For this review, take the finished solid that the model builds, in its own axes (mm). Coordinates: 2 decimals unless noted, no trailing zeros. Loops run counter-clockwise (first coordinate to the right, second up) from the corner with the lowest first, then second, coordinate; pieces in that order, holes last. Notation, with made-up numbers: (20, 64) -> (69, 64) arc R19 cw to (69, 95) -> close; hole circle Ø2 at (55.25, 64). An arc over 180 degrees is marked (long way). One line per item, written item: value.
from build123d import *

# Parameters (mm, degrees)
CROQUIS1_W              = 111
CROQUIS1_H              = 86.5
CROQUIS1_W_2            = 7.783251258
CROQUIS1_H_2            = 10.118226634
SALIENTE_EXTRUIR1_DEPTH = 5
CROQUIS3_W              = 111
CROQUIS3_H              = 5
SALIENTE_EXTRUIR2_DEPTH = 6


with BuildPart() as part:
    # Croquis1 → Saliente-Extruir1 (new body)
    with BuildSketch(Plane.XY):
        with Locations((50.205582562, 38.585714286)):
            Rectangle(CROQUIS1_W, CROQUIS1_H)
        Polygon((-1.339906851, 59.600947476), (4.653483533, 65.703308594), (73.52298758, 65.703308594), (73.52298758, 59.600947476), (6.614956749, 59.600947476), (6.614956749, 17.756185524), (81.586821915, 17.756185524), (81.586821915, 11), (6.614956749, 11), (-1.339906851, 11), align=None, mode=Mode.SUBTRACT)
        Polygon((29.151946634, 43.268500853), (37.324360454, 43.268500853), (37.324360454, 51.311193819), (61.582160207, 51.311193819), (61.582160207, 25.756185524), (37.324360454, 25.756185524), (37.324360454, 30.945019695), (29.151946634, 30.945019695), align=None, mode=Mode.SUBTRACT)
        with Locations((73.516478802, 50.815298841)):
            Rectangle(CROQUIS1_W_2, CROQUIS1_H_2, mode=Mode.SUBTRACT)
    extrude(amount=SALIENTE_EXTRUIR1_DEPTH)

    # Croquis3 → Saliente-Extruir2 (add)
    with BuildSketch(Plane(origin=(0, 81.835714286, 0), x_dir=(1, 0, 0), z_dir=(0, 1, 0))):
        with Locations((50.205582562, -2.5)):
            Rectangle(CROQUIS3_W, CROQUIS3_H)
    extrude(amount=SALIENTE_EXTRUIR2_DEPTH)


solid = part.part
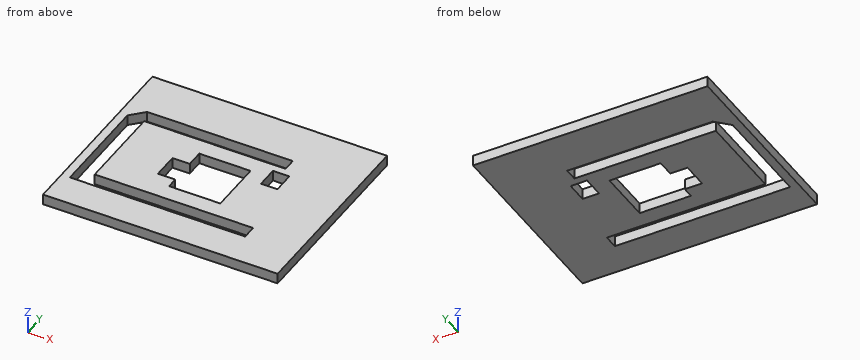
1. Take a section at D-D, the plane y = 23. Give the boundary of the cut face in (x, z).
Return value:
outline: (-5.29, 0) -> (-1.34, 0) -> (-1.34, 5) -> (-5.29, 5) -> close; (6.61, 0) -> (105.71, 0) -> (105.71, 5) -> (6.61, 5) -> close
2. Take a section at B-B, the plane x = 43.5. Give the boundary of the cut face in (y, z).
Return value:
outline: (-4.66, 0) -> (11, 0) -> (11, 5) -> (-4.66, 5) -> close; (17.76, 0) -> (25.76, 0) -> (25.76, 5) -> (17.76, 5) -> close; (51.31, 0) -> (59.6, 0) -> (59.6, 5) -> (51.31, 5) -> close; (65.7, 0) -> (87.84, 0) -> (87.84, 5) -> (65.7, 5) -> close
3. To check wall thickness, follow probe 1 along Y at (x, z) = (65.5, 0.3); probe 2 along Y at (x, z) = (41.5, 3.65); probe 3 along Y at (x, z) = (72, 1.5). State the ranges of each line that lie inside material, in increasing order. Write a range as from..to.
Return value:
probe 1: y = -4.66..11, 17.76..59.6, 65.7..87.84
probe 2: y = -4.66..11, 17.76..25.76, 51.31..59.6, 65.7..87.84
probe 3: y = -4.66..11, 17.76..45.76, 55.87..59.6, 65.7..87.84
4. Take a section at C-C, the plane z = 2.4. Give the boundary of the cut face in (x, y), and give its area (3 significant figures).
Return value:
outline: (-5.29, -4.66) -> (105.71, -4.66) -> (105.71, 87.84) -> (-5.29, 87.84) -> close; hole (-1.34, 11) -> (81.59, 11) -> (81.59, 17.76) -> (6.61, 17.76) -> (6.61, 59.6) -> (73.52, 59.6) -> (73.52, 65.7) -> (4.65, 65.7) -> (-1.34, 59.6) -> close; hole (29.15, 30.95) -> (37.32, 30.95) -> (37.32, 25.76) -> (61.58, 25.76) -> (61.58, 51.31) -> (37.32, 51.31) -> (37.32, 43.27) -> (29.15, 43.27) -> close; hole (69.62, 45.76) -> (77.41, 45.76) -> (77.41, 55.87) -> (69.62, 55.87) -> close
area: 8,140 mm2
5. Take a section at A-A, the plane y = 41. Give the boundary of the cut face in (x, z).
Return value:
outline: (-5.29, 0) -> (-1.34, 0) -> (-1.34, 5) -> (-5.29, 5) -> close; (6.61, 0) -> (29.15, 0) -> (29.15, 5) -> (6.61, 5) -> close; (61.58, 0) -> (105.71, 0) -> (105.71, 5) -> (61.58, 5) -> close
